Part model, mm, in its own coordinate system. Give positions to 0.01 mm unless a question says otherwise; leave off trailing zeros. Write each loop counter-clockwise with the first axis right and the second up, starting at its lowest first coordinate (ties: lowest second). Pieces come first, ordered by that corner, then holes. Notation, with made-up numbers: (26.25, 69.25) - (30.25, 69.25) arc R25 ccw to (30.25, 81.25) - close; hole circle Ø4 at (-13.5, 73). An arc over 180 degrees is marked (long way). Answer in a Markdown table with one row per item. Add a question column.
1. Pull direction Y, two halves, no side cores. Call faces 1 (the cylindrical face through (24.43, 24.4, 4.56)), 2 (the cylindrical face through (-13.277, -18.449, 4.437)), 3 (the cylindrical face through (24.4, -24.43, 4.56)), 4 (the cylindrical face through (19.885, -19.784, 4.437)): released by +Y, released by -Y, zero draft, split by the parting line, or undercut.
2. Probe line 1 along Y through (x, z) = (20.8, 6.25); line 2 along Y through (x, z) = (-14.5, 6); line 3 along X through (y, z) = (-19.5, 7.75). List the from-to ranges inside material, lowest first.
3. Band-saw the part on D-D on y = 20.8. Write the cut outline in (x, z).
4. Band-saw the part on B-B on z = 7. State how many separate pieces and enclosed holes the cut face has, plus the area to 3 significant figures.
5. Band-saw the part on A-A on x = 0. Write the cut outline in (y, z), plus the area to 3 significant figures.
6. Band-saw the part on C-C on y = 14.5. Write the cut outline in (x, z), plus the area to 3 significant figures.
Autodesk Inventor part; units mm, degrees
ref_plane "YZ Plane" through (0, 0, 0) normal (1, 0, 0) x (0, 1, 0)
ref_plane "XZ Plane" through (0, 0, 0) normal (0, 1, 0) x (-1, 0, 0)
ref_plane "XY Plane" through (0, 0, 0) normal (0, 0, 1) x (1, 0, 0)
sketch "Sketch1" plane through (0, 0, 0) normal (0, 0, 1) x (1, 0, 0)
  line L0 (-25, 25) -> (25, 25)
  line L1 (25, 25) -> (25, -25)
  line L2 (25, -25) -> (-25, -25)
  line L3 (-25, -25) -> (-25, 25)
  line L4 (-25, 25) -> (25, -25) construction
  line L5 (25, 25) -> (-25, -25) construction
  circle A0 centre (0, 0) radius 16
  circle A1 centre (-20.8, -14.5) radius 2.65
  circle A2 centre (-14.5, -20.8) radius 2.65
  circle A3 centre (-20.8, 14.5) radius 2.65
  circle A4 centre (20.8, -14.5) radius 2.65
  circle A5 centre (20.8, 14.5) radius 2.65
  circle A6 centre (-14.5, 20.8) radius 2.65
  circle A7 centre (14.5, -20.8) radius 2.65
  circle A8 centre (14.5, 20.8) radius 2.65
  dimension "d0" = 50
  dimension "d1" = 50
  dimension "d2" = 32
  dimension "d5" = 5.3
  dimension "d6" = 4.2
  dimension "d8" = 10.5
  dimension "d11" = 29
  dimension "d14" = 41.6
extrude "Extrusion1" add sketch "Sketch1" along normal blind 9
fillet "Fillet1" radius 2 4 edges at (-25, 25, 4.5) (25, 25, 4.5) (-25, -25, 4.5) (25, -25, 4.5)
sketch "Sketch2" plane through (0, 0, 9) normal (0, 0, 1) x (1, 0, 0)
  arc A0 (23, -25) -> (25, -23) centre (23, -23) ccw
  line L0 (25, -23) -> (25, 23)
  arc A1 (25, 23) -> (23, 25) centre (23, 23) ccw
  line L1 (23, 25) -> (-23, 25)
  arc A2 (-23, 25) -> (-25, 23) centre (-23, 23) ccw
  line L2 (-25, 23) -> (-25, -23)
  arc A3 (-25, -23) -> (-23, -25) centre (-23, -23) ccw
  line L3 (-23, -25) -> (23, -25)
  circle A4 centre (14.5, 20.8) radius 2.65
  circle A5 centre (-14.5, 20.8) radius 2.65
  circle A6 centre (14.5, -20.8) radius 2.65
  circle A7 centre (20.8, 14.5) radius 2.65
  circle A8 centre (20.8, -14.5) radius 2.65
  circle A9 centre (-20.8, 14.5) radius 2.65
  circle A10 centre (-14.5, -20.8) radius 2.65
  circle A11 centre (-20.8, -14.5) radius 2.65
  circle A12 centre (0, 0) radius 16
  line L4 (21, -21) -> (-21, -21)
  line L5 (-21, -21) -> (-21, 21)
  line L6 (-21, 21) -> (21, 21)
  line L7 (21, 21) -> (21, -21)
  line L8 (21, -21) -> (-21, 21) construction
  line L9 (-21, -21) -> (21, 21) construction
  circle A13 centre (-28.6, 21.06) radius 1.55
  dimension "d18" = 42
  dimension "d19" = 42
hole "Hole1" at (-21, 21, 9) at (21, 21, 9) at (21, -21, 9) at (-21, -21, 9) direction (0, 0, -1) diameter 3.3 end through all both
properties part number "20_IM_LED_holder"
Values:
| question | item | result |
|---|---|---|
| 1 | face 1 | released by +Y |
| 1 | face 2 | undercut |
| 1 | face 3 | released by -Y |
| 1 | face 4 | undercut |
| 2 | line 1 | y = -25 to -22.64, -19.36 to -17.15, -11.85 to 11.85, 17.15 to 19.36, 22.64 to 25 |
| 2 | line 2 | y = -25 to -23.45, -18.15 to -6.76, 6.76 to 18.15, 23.45 to 25 |
| 2 | line 3 | x = -25 to -21.69, -20.31 to -16.81, -12.19 to 12.19, 16.81 to 20.31, 21.69 to 25 |
| 3 | outline | (-25, 0) - (-22.64, 0) - (-22.64, 9) - (-25, 9) - close; (-19.36, 0) - (-17.15, 0) - (-17.15, 9) - (-19.36, 9) - close; (-11.85, 0) - (11.85, 0) - (11.85, 9) - (-11.85, 9) - close; (17.15, 0) - (19.36, 0) - (19.36, 9) - (17.15, 9) - close; (22.64, 0) - (25, 0) - (25, 9) - (22.64, 9) - close |
| 4 | separate pieces | 1 |
| 4 | enclosed holes | 13 |
| 4 | area | 1,480 mm² |
| 5 | outline | (-25, 0) - (-16, 0) - (-16, 9) - (-25, 9) - close; (16, 0) - (25, 0) - (25, 9) - (16, 9) - close |
| 5 | area | 162 mm² |
| 6 | outline | (-25, 0) - (-23.45, 0) - (-23.45, 9) - (-25, 9) - close; (-18.15, 0) - (-6.76, 0) - (-6.76, 9) - (-18.15, 9) - close; (6.76, 0) - (18.15, 0) - (18.15, 9) - (6.76, 9) - close; (23.45, 0) - (25, 0) - (25, 9) - (23.45, 9) - close |
| 6 | area | 233 mm² |
